from build123d import *

# Parameters (mm, degrees)
F1_DEPTH = 4
F3_D     = 2
F4_R     = 1
F5_R     = 1
F7_DEPTH = 6


with BuildPart() as f1:
    # F0 (on Front) → F1 (new body)
    with BuildSketch(Plane.XZ):
        with BuildLine():
            Line((4.3, 0), (4.3, 4.35))
            Line((4.3, 4.35), (-5.7, 4.35))
            ThreePointArc((-5.7, 4.35), (-6.407107, 4.057107), (-6.7, 3.35))
            Line((-6.7, 3.35), (-6.7, 2.5))
            ThreePointArc((-6.7, 2.5), (-6.992893, 1.792893), (-7.7, 1.5))
            Line((-7.7, 1.5), (-25, 1.5))
            ThreePointArc((-25, 1.5), (-25.378059, 1.425782), (-25.7, 1.214143))
            Line((-25.7, 1.214143), (-25.7, -1.214143))
            ThreePointArc((-25.7, -1.214143), (-25.378059, -1.425782), (-25, -1.5))
            Line((-25, -1.5), (-7.7, -1.5))
            ThreePointArc((-7.7, -1.5), (-6.992893, -1.792893), (-6.7, -2.5))
            Line((-6.7, -2.5), (-6.7, -3.35))
            ThreePointArc((-6.7, -3.35), (-6.407107, -4.057107), (-5.7, -4.35))
            Line((-5.7, -4.35), (4.3, -4.35))
            Line((4.3, -4.35), (4.3, 0))
        make_face()
        with BuildLine():
            ThreePointArc((-2.034699, -1.85), (-2.75, 0), (-2.034699, 1.85))
            Line((-2.034699, 1.85), (2.034699, 1.85))
            ThreePointArc((2.034699, 1.85), (2.75, 0), (2.034699, -1.85))
            Line((2.034699, -1.85), (-2.034699, -1.85))
        make_face(mode=Mode.SUBTRACT)
    extrude(amount=F1_DEPTH)

    # F3 (through all)
    with Locations(Plane.XY.offset(4.35)):
        with Locations((-23, -2)):
            Hole(F3_D / 2)

    # F4
    f4_edges = [f1.edges().sort_by_distance(p)[0] for p in [
        (4.3, -2, 4.35),
    ]]
    fillet(f4_edges, radius=F4_R)

    # F5
    f5_edges = [f1.edges().sort_by_distance(p)[0] for p in [
        (4.3, -2, -4.35),
    ]]
    fillet(f5_edges, radius=F5_R)

    # F6 (on face) → F7 (join)
    with BuildSketch(Plane.XZ.offset(4)):
        with BuildLine():
            ThreePointArc((-2.580698, 3.25), (-4.15, 0), (-2.580698, -3.25))
            Line((-2.580698, -3.25), (2.580698, -3.25))
            ThreePointArc((2.580698, -3.25), (4.15, 0), (2.580698, 3.25))
            Line((2.580698, 3.25), (-2.580698, 3.25))
        make_face()
        with BuildLine():
            Line((2.034699, -1.85), (-2.034699, -1.85))
            ThreePointArc((-2.034699, -1.85), (-2.75, 0), (-2.034699, 1.85))
            Line((-2.034699, 1.85), (2.034699, 1.85))
            ThreePointArc((2.034699, 1.85), (2.75, 0), (2.034699, -1.85))
        make_face(mode=Mode.SUBTRACT)
    extrude(amount=F7_DEPTH)


solid = f1.part
Source: CAD feature listing. Evaluate the final solid. Frame: model axes, mm. A direction names the side the tool comes from. Round coordinates to 2 decimals unless told otherwise and drop trailing zeros. Loops run counter-clockwise (first coordinate to the right, second up) from the corner with the lowest first, then second, coordinate; pieces in that order, holes last. Notation, with made-up numbers: (41.5, 9) -> (84.5, 9) arc R24 ccw to (84.5, 45) -> close; hole circle Ø8 at (76, 19.25). An arc over 180 degrees is marked (long way). Answer as a JSON object with one key per item and string values. Group by question number.
Q1. Mould query, pull axis X, two halves, no side actions, for faces 5 (the cylindrical face through (4.15, -6.96, -0.05)), 6 (the flat face through (-11, -4, 0)), 7 (the cylindrical face through (-22, -2, 0)), 8 (the cylindrical face through (-6.985, -1.972, 1.801)). Classes: pulls with the +X half, pulls with the -X half, needs draft (parallel to the pull), parting line crosses it, or undercut.
Q2. Section query A-A (y = -2). Output: boundary loops of the cut face in (x, z), plus the area to 3 significant figures.
Q3. Access query for faces 1 (the flat face through (-16, -2, -1.5)), 2 (the flat face through (0, -5, 1.85)), 3 (the flat face through (-16, -2, 1.5)), 4 (the flat face through (4.3, -2, 0)). Directions: +Z, -Z, +X, -X, +Y, -Y. A direction counts if a zero-diameter tool reaches every point of the face in a straight line with its end or side. Return the directions, or none.
Q4. Ray query, line 1 (Z direction, x = 1.5, y = -0.5); line 2 (Y direction, x = -23, z = 0.35); line 3 (X direction, y = -1.5, z = 0.5). Return the intervals inside material, ascending. Write a range as from..to.
Q5. Contact query for flat-ended pins moving along their axis: P1, Ø3, axis at x = -20.5, y = -2, coming from the -Z side; P2, Ø1.6, axis at x = -23, y = -2, coming from the -Z side; P3, Ø4.5, axis at x = 0, y = -6.5, coming from the -Z side; P4, Ø0.9, axis at y = -3, z = 3, coming from the -X side. Output: stop coordinate, or through.
Q6. Section query B-B (x = -23). Output: boundary loops of the cut face in (y, z), plus the area to 3 significant figures.
Q7. Section query D-D (y = -8.25). Output: boundary loops of the cut face in (x, z), plus the area to 3 significant figures.
Q8. Section query C-C (z = -0.25). Output: boundary loops of the cut face in (x, y), plus the area to 3 significant figures.
Completed:
{
 "1": {"face 5": "pulls with the +X half", "face 6": "needs draft", "face 7": "undercut", "face 8": "pulls with the -X half"},
 "2": {"outline": "(-25.7, -1.21) arc R1 ccw to (-25, -1.5) -> (-24, -1.5) -> (-24, 1.5) -> (-25, 1.5) arc R1 ccw to (-25.7, 1.21) -> close; (-22, -1.5) -> (-7.7, -1.5) arc R1 cw to (-6.7, -2.5) -> (-6.7, -3.35) arc R1 ccw to (-5.7, -4.35) -> (3.3, -4.35) arc R1 ccw to (4.3, -3.35) -> (4.3, 3.35) arc R1 ccw to (3.3, 4.35) -> (-5.7, 4.35) arc R1 ccw to (-6.7, 3.35) -> (-6.7, 2.5) arc R1 cw to (-7.7, 1.5) -> (-22, 1.5) -> close; hole (-2.03, -1.85) -> (2.03, -1.85) arc R2.75 ccw to (2.03, 1.85) -> (-2.03, 1.85) arc R2.75 ccw to start", "area": "127 mm²"},
 "3": {"face 1": "-Z, -X, +Y, -Y", "face 2": "+Y, -Y", "face 3": "+Z, -X, +Y, -Y", "face 4": "+Z, -Z, +X, +Y, -Y"},
 "4": {"line 1": "-4.35..-1.85, 1.85..4.35", "line 2": "-4..-3, -1..0", "line 3": "-25.7..-23.87, -22.13..-2.7, 2.7..4.3"},
 "5": {"P1": "z = -1.5", "P2": "through", "P3": "z = -3.25", "P4": "x = -6.7"},
 "6": {"outline": "(-4, -1.5) -> (-3, -1.5) -> (-3, 1.5) -> (-4, 1.5) -> close; (-1, -1.5) -> (0, -1.5) -> (0, 1.5) -> (-1, 1.5) -> close", "area": "6.00 mm²"},
 "7": {"outline": "(-2.58, -3.25) -> (2.58, -3.25) arc R4.15 ccw to (2.58, 3.25) -> (-2.58, 3.25) arc R4.15 ccw to start; hole (-2.03, -1.85) -> (2.03, -1.85) arc R2.75 ccw to (2.03, 1.85) -> (-2.03, 1.85) arc R2.75 ccw to start", "area": "29.1 mm²"},
 "8": {"outline": "(-25.7, -4) -> (-4.14, -4) -> (-4.14, -10) -> (-2.74, -10) -> (-2.74, 0) -> (-25.7, 0) -> close; (2.74, -10) -> (4.14, -10) -> (4.14, -4) -> (4.3, -4) -> (4.3, 0) -> (2.74, 0) -> close; hole circle Ø2 at (-23, -2)", "area": "112 mm²"}
}
